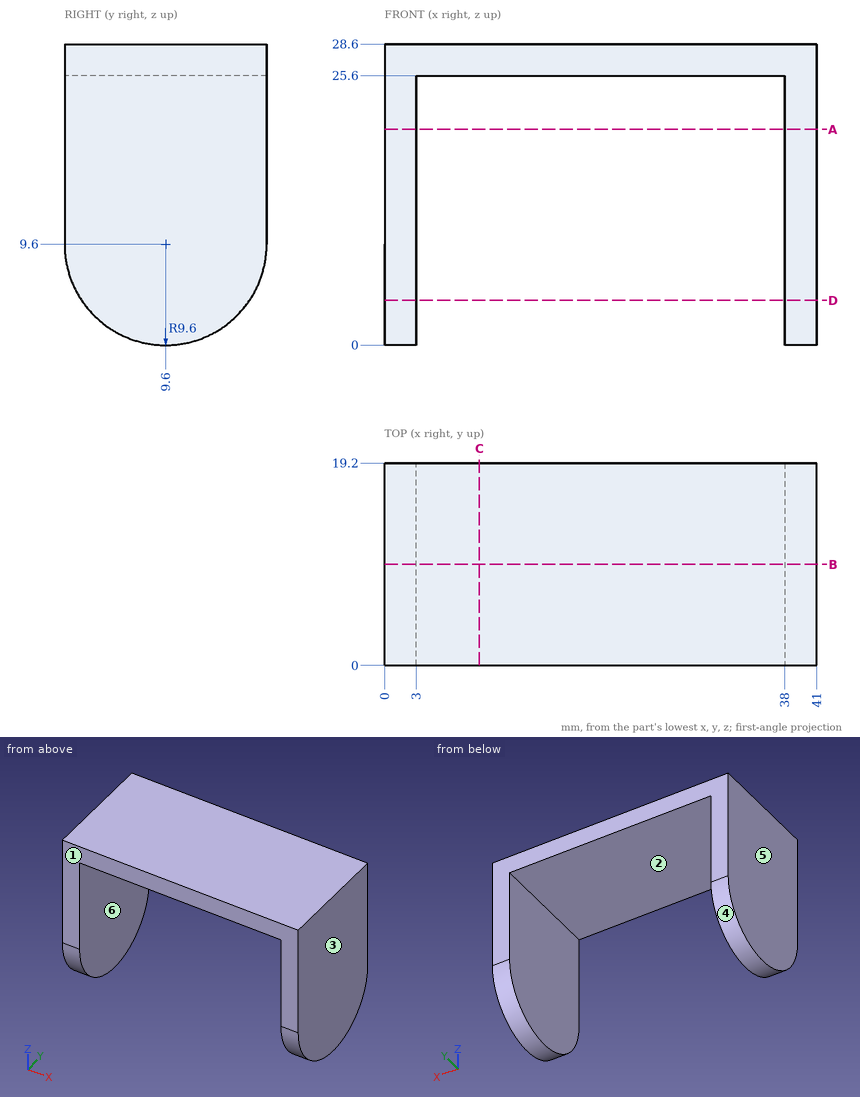
Here's the drawing with two shaded views (mm, measured from the low corner). I have some questions. A direction names the side the tool comes from. Coordinates: 2 decimals unless noted, no trailing zeros. Write each loop counter-clockwise with the first axis right and the second up, starting at its lowest first coordinate (ties: lowest second). Pieces come first, ordered by that corner, then holes. Notation, with made-up numbers: M 81.25,60 L 85.25,60 A30 ccw 85.25,85 Z; hole C 83,48.25 d6. An arc over 180 degrees is marked long. Answer as CSV lines item,"result".
Item 1: Imagine slicing it at A-A on z = 20.5. List the corners of the cut face in (x, y) for me, plus the area to 3 significant figures.
Geometry results:
outline,"M 0,0 L 3,0 L 3,19.2 L 0,19.2 Z; M 38,0 L 41,0 L 41,19.2 L 38,19.2 Z"
area,"115 mm2"
Item 2: I'm going to push a flat-ended pin straight in: P1, Ø1, axis at x = 5, z = 19, coming from the -Y side. Where does the tip first touch, or does it pass through?
Geometry results:
P1,"passes through"
Item 3: On a 3-axis mill with a long thin cutter (end or side, diameter ignored), from which of +Z, -Z, +X, -X, +Y, -Y can I reach the whole of each face in a straight line? I mean the marked faces 1 and 2. Say none if no direction works.
Geometry results:
face 1,"+Z, -Z, +X, -X, -Y"
face 2,"-Z, +Y, -Y"
Item 4: Please list where these lines run through material, in increasing order: line 1 along X through (y, z) = (14, 12.5); line 2 along Z through (x, y) = (11.5, 6.5); line 3 along Z through (x, y) = (39.5, 9.5).
Geometry results:
line 1,"x = 0 to 3, 38 to 41"
line 2,"z = 25.6 to 28.6"
line 3,"z = 0 to 28.6"
Item 5: Imagine slicing it at B-B on y = 9.6. List the corners of the cut face in (x, z) for me, plus the area to 3 significant figures.
Geometry results:
outline,"M 0,0 L 3,0 L 3,25.6 L 38,25.6 L 38,0 L 41,0 L 41,28.6 L 0,28.6 Z"
area,"277 mm2"
Item 6: We'd pull the mould along X, two halves only. Please class the marked faces 3, 4, 5 and 6: +X half, -X half, draft (parallel to the pull), parting line (faces both ways), or undercut.
Geometry results:
face 3,"+X half"
face 4,"draft"
face 5,"-X half"
face 6,"undercut"
Item 7: Imagine slicing it at C-C on x = 9. List the corners of the cut face in (y, z) for me, plus the area to 3 significant figures.
Geometry results:
outline,"M 0,25.6 L 19.2,25.6 L 19.2,28.6 L 0,28.6 Z"
area,"57.6 mm2"
Item 8: Imagine slicing it at D-D on z = 4.25. List the corners of the cut face in (x, y) for me.
Geometry results:
outline,"M 0,1.63 L 3,1.63 L 3,17.57 L 0,17.57 Z; M 38,1.63 L 41,1.63 L 41,17.57 L 38,17.57 Z"
